from build123d import *

# Parameters (mm, degrees)
SZKIC1_W                    = 15
SZKIC1_H                    = 14
DODANIE_WYCI_GNI_CIE1_DEPTH = 13.5
SZKIC2_R                    = 2.625
WYTNIJ_WYCI_GNI_CIE1_DEPTH  = 15
ZAOKR_GLENIE1_R             = 3.5
WYTNIJ_WYCI_GNI_CIE2_DEPTH  = 15
ZAOKR_GLENIE2_R             = 3
SZKIC4_R                    = 5.5
WYTNIJ_WYCI_GNI_CIE3_DEPTH  = 3


with BuildPart() as part:
    # Szkic1 → Dodanie-wyciągnięcie1 (new body)
    with BuildSketch(Plane(origin=(0, 0, 0), x_dir=(1, 0, 0), z_dir=(0, 1, 0))):
        Rectangle(SZKIC1_W, SZKIC1_H)
    extrude(amount=DODANIE_WYCI_GNI_CIE1_DEPTH)

    # Szkic2 → Wytnij-wyciągnięcie1 (cut)
    with BuildSketch(Plane.XY.offset(7)):
        with Locations((0, 8.75)):
            Circle(SZKIC2_R)
    extrude(amount=-WYTNIJ_WYCI_GNI_CIE1_DEPTH, mode=Mode.SUBTRACT)

    # Zaokrąglenie1
    zaokr_glenie1_edges = [part.edges().sort_by_distance(p)[0] for p in [
        (-7.5, 13.5, 0),
    ]]
    fillet(zaokr_glenie1_edges, radius=ZAOKR_GLENIE1_R)

    # Szkic3 → Wytnij-wyciągnięcie2 (cut)
    with BuildSketch(Plane.XY.offset(7)):
        Polygon((0.95, 13.5), (7.5, 11), (7.5, 13.5), align=None)
    extrude(amount=-WYTNIJ_WYCI_GNI_CIE2_DEPTH, mode=Mode.SUBTRACT)

    # Zaokrąglenie2
    zaokr_glenie2_edges = [part.edges().sort_by_distance(p)[0] for p in [
        (0.95, 13.5, 0),
    ]]
    fillet(zaokr_glenie2_edges, radius=ZAOKR_GLENIE2_R)

    # Szkic4 → Wytnij-wyciągnięcie3 (cut)
    with BuildSketch(Plane.XZ):
        with Locations(Location((0, 0, 0), (0, 0, 270))):
            Circle(SZKIC4_R)
    extrude(amount=-WYTNIJ_WYCI_GNI_CIE3_DEPTH, mode=Mode.SUBTRACT)


solid = part.part
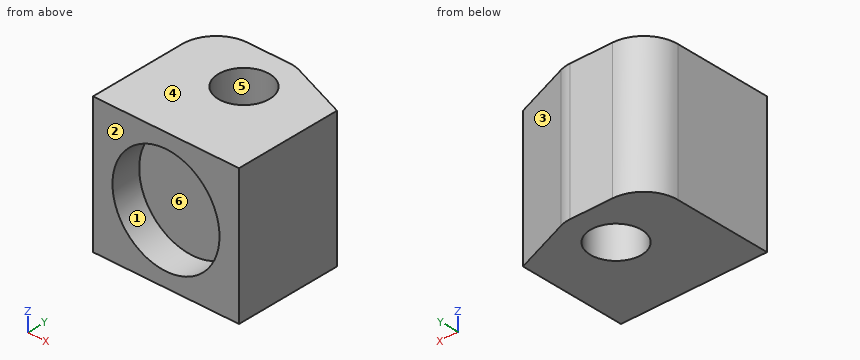
Can you work these out from the model? Positions are in its coordinate system, mm. Face numbers are marked on the shaded views. A direction names the side the tool comes from. Give positions to 0.01 mm unless a question says otherwise; leave off trailing zeros. Loops run counter-clockwise (first coordinate to the right, second up) from the corner with the lowest first, then second, coordinate; pieces in that order, holes last. Notation, with made-up numbers: (89.25, 9.5) -> (131.25, 9.5) arc R8 cw to (131.25, 16.5) -> close; hole circle Ø5 at (65, 35.5). An arc over 180 degrees is marked (long way). Return JSON: item names as keys, results as strings.
Q1. On a 3-axis mill with a long thin cutter (end or side, diameter ignored), from which of +Z, -Z, +X, -X, +Y, -Y can I reach the whole of each face in a straight line? I mean the marked faces 1 and 2. Say none if no direction works.
Checks:
{"face 1": "-Y", "face 2": "+Z, -Z, +X, -X, -Y"}
Q2. For pin 1 Ø3.5 at (x, z) = (2.5, 2) entering from -Y, with a flat end and sliding along its axis, tell me the tip position at first contact or that it passes through.
Checks:
{"pin 1": "stops at y = 3"}
Q3. I want a section at A-A, the plane y = 8.75. List the corners of the cut face in (x, z) for me (3 decimals), then the cut area to 4 significant figures.
Checks:
{"outline": "(-7.5, -7) -> (-2.625, -7) -> (-2.625, 7) -> (-7.5, 7) -> close; (2.625, -7) -> (7.5, -7) -> (7.5, 7) -> (2.625, 7) -> close", "area": "136.5 mm2"}
Q4. I want a section at D-D, the plane x = 4. List the corners of the cut face in (y, z) for me.
Checks:
{"outline": "(0, -7) -> (12.34, -7) -> (12.34, 7) -> (0, 7) -> (0, 3.77) -> (3, 3.77) -> (3, -3.77) -> (0, -3.77) -> close"}
Q5. I need wall thicknesses on probe 1 along Y at (x, z) = (0, 2.5) (3 decimals); probe 2 along X at (y, z) = (1.85, 0); probe 3 along X at (y, z) = (1.75, 3). Which ranges of each line are inside material? Lowest first, please.
Checks:
{"probe 1": "y = 3 to 6.125, 11.375 to 13.5", "probe 2": "x = -7.5 to -5.5, 5.5 to 7.5", "probe 3": "x = -7.5 to -4.61, 4.61 to 7.5"}
Q6. I want a section at B-B, the plane z = 0. List the corners of the cut face in (x, y) for me (3 decimals), then the cut area to 3 significant figures.
Checks:
{"outline": "(-7.5, 0) -> (-5.5, 0) -> (-5.5, 3) -> (5.5, 3) -> (5.5, 0) -> (7.5, 0) -> (7.5, 11) -> (1.467, 13.303) arc R3 ccw to (0.397, 13.5) -> (-4, 13.5) arc R3.5 ccw to (-7.5, 10) -> close; hole circle Ø5.25 at (0, 8.75)", "area": "137 mm2"}
Q7. We'd pull the mould along X, two halves only. Please class the marked faces 3, 4, 5 and 6: released by +X, released by -X, zero draft, split by the parting line, or undercut.
Checks:
{"face 3": "released by +X", "face 4": "zero draft", "face 5": "undercut", "face 6": "undercut"}
Q8. I want a section at C-C, the plane x = 0. List the corners of the cut face in (y, z) for me (3 decimals), then the cut area to 3 significant figures.
Checks:
{"outline": "(0, -7) -> (6.125, -7) -> (6.125, 7) -> (0, 7) -> (0, 5.5) -> (3, 5.5) -> (3, -5.5) -> (0, -5.5) -> close; (11.375, -7) -> (13.5, -7) -> (13.5, 7) -> (11.375, 7) -> close", "area": "82.5 mm2"}
